Verification items for the finished model (mm, model axes). Face numbers are marked on the shaded views. A direction names the side the tool comes from. Coordinates: 2 decimals unless noted, no trailing zeros. Write each loop counter-clockwise with the first axis right and the second up, starting at its lowest first coordinate (ties: lowest second). Pieces come first, ordered by that corner, then holes. Notation, with made-up numbers: (-16, 76) -> (43, 76) arc R11 ccw to (43, 92) -> close; hole circle Ø10 at (38.25, -6.5). An arc over 180 degrees is marked (long way). Write each question's results on one line, items separated by ' | '. Start each with the question number.
from build123d import *

# Parameters (mm, degrees)
BOSS_EXTRUDE1_DEPTH      = 12.7
BOSS_EXTRUDE1_DEPTH_BACK = 12.7
SKETCH1_R                = 4.445
SKETCH9_W                = 30.48
SKETCH9_H                = 35.052
CUT_EXTRUDE6_DEPTH       = 60.613097773
BOSS_EXTRUDE3_DEPTH      = 12.7
SKETCH11_W               = 5.350768363
SKETCH11_H               = 57.15
CUT_EXTRUDE7_DEPTH       = 75.08914513
SKETCH12_W               = 30.48
SKETCH12_H               = 19.05
CUT_EXTRUDE8_DEPTH       = 89.211973463
SKETCH14_R               = 1.6
CUT_EXTRUDE9_DEPTH       = 75.795998583
SKETCH15_R               = 3.429
CUT_EXTRUDE10_DEPTH      = 75.795998583
CUT_EXTRUDE11_DEPTH      = 2.778125
F_6_CLEARANCE_HOLE1_D    = 3.7973
SKETCH25_W               = 89.81357484
SKETCH25_H               = 39.457269438
CUT_EXTRUDE14_DEPTH      = 67.031594151


with BuildPart() as part:
    # Sketch1 → Boss-Extrude1 (new, two sides: drawn at the far end of the back side and taken through both)
    with BuildSketch(Plane.XY.offset(-BOSS_EXTRUDE1_DEPTH_BACK)):
        with BuildLine():
            Line((-26.940768363, -17.415768363), (-26.940768363, 39.734231637))
            Line((-26.940768363, 39.734231637), (26.940768363, 39.734231637))
            Line((26.940768363, 39.734231637), (26.940768363, -17.415768363))
            ThreePointArc((26.940768363, -17.415768363), (36.465768363, -26.940768363), (26.940768363, -36.465768363))
            Line((26.940768363, -36.465768363), (-26.940768363, -36.465768363))
            ThreePointArc((-26.940768363, -36.465768363), (-36.465768363, -26.940768363), (-26.940768363, -17.415768363))
        make_face()
        with Locations((-26.940768363, -26.940768363)):
            Circle(SKETCH1_R, mode=Mode.SUBTRACT)
        with Locations((26.940768363, -26.940768363)):
            Circle(SKETCH1_R, mode=Mode.SUBTRACT)
    extrude(amount=BOSS_EXTRUDE1_DEPTH + BOSS_EXTRUDE1_DEPTH_BACK)

    # Sketch9 → Cut-Extrude6 (cut, through all)
    with BuildSketch(Plane.XY.offset(12.7)):
        with Locations((0, 22.208231637)):
            Rectangle(SKETCH9_W, SKETCH9_H)
    extrude(amount=-CUT_EXTRUDE6_DEPTH, mode=Mode.SUBTRACT)

    # Sketch10 → Boss-Extrude3 (add)
    with BuildSketch(Plane.XY.offset(12.7)):
        Polygon((-26.940768363, 39.734231637), (-26.940768363, -1.667768363), (26.940768363, -1.667768363), (26.940768363, 39.734231637), (15.24, 39.734231637), (15.24, 4.682231637), (-15.24, 4.682231637), (-15.24, 39.734231637), align=None)
    boss_extrude3 = extrude(amount=BOSS_EXTRUDE3_DEPTH)

    # Mirror4: Boss-Extrude3 across plane
    add(boss_extrude3.mirror(Plane.XY))

    # Sketch11 → Cut-Extrude7 (cut, through all)
    with BuildSketch(Plane.XY.offset(25.4)):
        with Locations((-24.265384181, 11.159231637)):
            Rectangle(SKETCH11_W, SKETCH11_H)
    cut_extrude7 = extrude(amount=-CUT_EXTRUDE7_DEPTH, mode=Mode.SUBTRACT)

    # Mirror5: Cut-Extrude7 across plane
    add(cut_extrude7.mirror(Plane(origin=(0, 0, 0), x_dir=(0, 0, 1), z_dir=(1, 0, 0))), mode=Mode.SUBTRACT)

    # Sketch12 → Cut-Extrude8 (cut, through all)
    with BuildSketch(Plane.XZ.offset(36.465768363)):
        Rectangle(SKETCH12_W, SKETCH12_H)
    extrude(amount=-CUT_EXTRUDE8_DEPTH, mode=Mode.SUBTRACT)

    # Sketch14 → Cut-Extrude9 (cut, through all)
    with BuildSketch(Plane.ZY.offset(21.59)):
        with Locations(Location((-18.4, 22.462231637, 0), (0, 0, 90))):
            Circle(SKETCH14_R)
    cut_extrude9 = extrude(amount=-CUT_EXTRUDE9_DEPTH, mode=Mode.SUBTRACT)

    # Mirror6: Cut-Extrude9 across plane
    add(cut_extrude9.mirror(Plane.XY), mode=Mode.SUBTRACT)

    # Sketch15 → Cut-Extrude10 (cut, through all)
    with BuildSketch(Plane(origin=(21.59, 0, 0), x_dir=(0, 0, -1), z_dir=(1, 0, 0))):
        with Locations(Location((0, 22.462231637, 0), (0, 0, 90))):
            Circle(SKETCH15_R)
    extrude(amount=-CUT_EXTRUDE10_DEPTH, mode=Mode.SUBTRACT)

    # Sketch18 → Cut-Extrude11 (cut)
    with BuildSketch(Plane(origin=(0, 4.682231637, 0), x_dir=(1, 0, 0), z_dir=(0, 1, 0))):
        Polygon((4.064, 21.396351494), (0, 23.742702988), (-4.064, 21.396351494), (-4.064, 16.703648506), (0, 14.357297012), (4.064, 16.703648506), align=None)
    cut_extrude11 = extrude(amount=-CUT_EXTRUDE11_DEPTH, mode=Mode.SUBTRACT)

    # Mirror7: Cut-Extrude11 across plane
    add(cut_extrude11.mirror(Plane.XY), mode=Mode.SUBTRACT)

    # 6 Clearance Hole1 (through all)
    with Locations(Plane(origin=(0, 1.904106637, 0), x_dir=(1, 0, 0), z_dir=(0, 1, 0))):
        with Locations((0, 19.05)):
            f_6_clearance_hole1 = Hole(F_6_CLEARANCE_HOLE1_D / 2)

    # Mirror8: 6 Clearance Hole1 across plane
    add(f_6_clearance_hole1.mirror(Plane.XY), mode=Mode.SUBTRACT)

    # Sketch25 → Cut-Extrude14 (cut, through all)
    with BuildSketch(Plane(origin=(0, 0, -12.7), x_dir=(-1, 0, 0), z_dir=(0, 0, -1))):
        with Locations((0.758793643, -21.396403082)):
            Rectangle(SKETCH25_W, SKETCH25_H)
    extrude(amount=-CUT_EXTRUDE14_DEPTH, mode=Mode.SUBTRACT)


solid = part.part
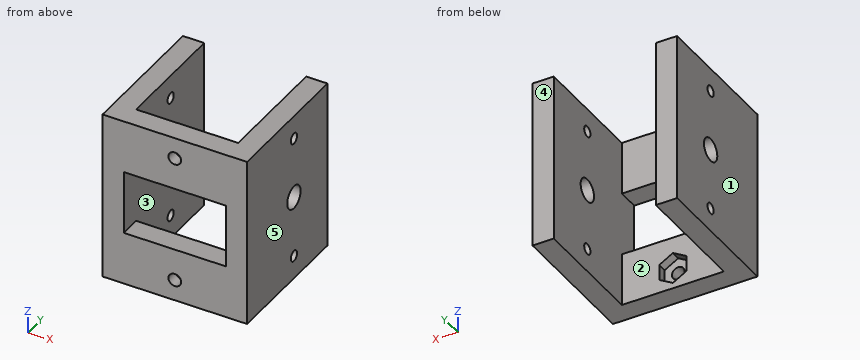
1. Sectioned sample at D-D on x = 18.5. Record the cut outline in (y, z).
2. Tool access check on the marked faces 1 and 2. Record the directions out of +Z, -Z, +X, -X, +Y, -Y that give a thin tool (end or side, any length) a straight path to the whole face; none if there is none.
3. Mould release check, pull along X, two halves, no side actions. Record for the marked faces 3, 4 and 5: +X half, -X half, draft (parallel to the pull), parting line (faces both ways), or undercut.
4. Sectioned sample at C-C on z = -19.05. Record the cut outline in (x, y), plus the area to 3 significant figures.
5. Sectioned sample at B-B on x = -13. Record the cut outline in (y, z) (3 decimals), plus the area to 3 significant figures.
6. Material ranges on probe 1 along Z at (x, y) = (0, 0) (3 decimals); probe 2 along X at (y, z) = (9.5, -8.5); probe 3 along Y at (x, z) = (20.25, 18.4), recorded low to high. Write a range as from..to.
7. Sectioned sample at A-A on y = 11. Record the cut outline in (x, z).
8. Depth check by flat-ended pin: pin 1 Ø2.5 at (x, z) = (-1, 19) entering from +Y; pin 2 Ø12.5 at (x, z) = (-1.5, 14.5) entering from +Y. Enter the tip coordinate at first touch or a pass-through.
Computed values:
1) outline: (-1.67, -25.4) -> (39.73, -25.4) -> (39.73, 25.4) -> (-1.67, 25.4) -> close; hole circle Ø6.86 at (22.46, 0); hole circle Ø3.2 at (22.46, -18.4); hole circle Ø3.2 at (22.46, 18.4)
2) face 1: +Z, -Z, -X, +Y, -Y | face 2: +Z, -Z, +Y
3) face 3: undercut | face 4: draft | face 5: +X half
4) outline: (-21.59, -1.67) -> (-1.9, -1.67) -> (-1.9, 1.9) -> (-4.06, 1.9) -> (-4.06, 4.68) -> (-15.24, 4.68) -> (-15.24, 21) -> (-21.59, 21) -> close; (-21.59, 23.92) -> (-15.24, 23.92) -> (-15.24, 39.73) -> (-21.59, 39.73) -> close; (1.9, -1.67) -> (21.59, -1.67) -> (21.59, 21) -> (15.24, 21) -> (15.24, 4.68) -> (4.06, 4.68) -> (4.06, 1.9) -> (1.9, 1.9) -> close; (15.24, 23.92) -> (21.59, 23.92) -> (21.59, 39.73) -> (15.24, 39.73) -> close | area: 646 mm^2
5) outline: (-1.668, -25.4) -> (4.682, -25.4) -> (4.682, -9.525) -> (-1.668, -9.525) -> close; (-1.668, 9.525) -> (4.682, 9.525) -> (4.682, 25.4) -> (-1.668, 25.4) -> close | area: 202 mm^2
6) probe 1: z = -25.4..-20.949, -17.151..-9.525, 9.525..17.151, 20.949..25.4 | probe 2: x = -21.59..-15.24, 15.24..21.59 | probe 3: y = -1.67..20.86, 24.06..39.73
7) outline: (-21.59, -25.4) -> (-15.24, -25.4) -> (-15.24, 25.4) -> (-21.59, 25.4) -> close; (15.24, -25.4) -> (21.59, -25.4) -> (21.59, 25.4) -> (15.24, 25.4) -> close
8) pin 1: stops at y = 1.9 | pin 2: stops at y = 4.68
